For this review, take the finished solid that the model builds, in its own axes (mm). Face numbers are marked on the shaded views. A direction names the side the tool comes from. Give positions to 0.01 mm unless a question says otherwise; leave off trailing zeros. Loops run counter-clockwise (first coordinate to the right, second up) from the corner with the lowest first, then second, coordinate; pieces in that order, holes last. Notation, with made-up numbers: (36, -0.5) - (92, -0.5) arc R13 cw to (92, 20.5) - close; hole circle Ø8 at (-13.75, -2). An arc over 180 degrees is marked (long way). Answer as CSV lines item,"result".
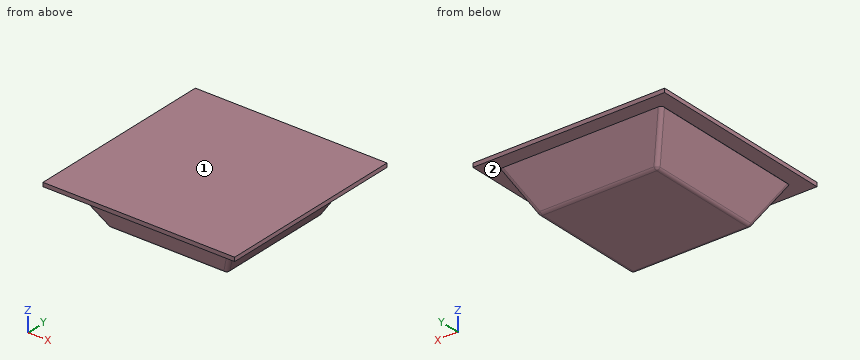
Solid Edge part; units mm, degrees
sketch "Sketch1" plane through (0, 0, 0) normal (0, 0, 1) x (1, 0, 0)
  line L0 (41, -41) -> (-41, -41)
  line L1 (-41, -41) -> (-41, 41)
  line L2 (-41, 41) -> (41, 41)
  line L3 (41, 41) -> (41, -41)
  dimension "D1" = 41
  dimension "D2" = 41
extrude "Protrusion1" add sketch "Sketch1" along normal blind 20
sketch "Sketch2" plane through (41, 0, 10) normal (1, 0, 0) x (0, 1, 0)
  line L0 (-41, 10) -> (-30, -10)
  line L1 (-30, -10) -> (30, -10)
  line L2 (30, -10) -> (41, 10)
  line L3 (-41, 10) -> (41, 10)
extrude "Cutout1" cut sketch "Sketch2" against normal through all flip side to cut
sketch "Sketch3" plane through (0, 0, 20) normal (0, 0, 1) x (0, 1, 0)
  line L0 (48.5, -48.5) -> (-48.5, -48.5)
  line L1 (-48.5, -48.5) -> (-48.5, 48.5)
  line L2 (-48.5, 48.5) -> (48.5, 48.5)
  line L3 (48.5, 48.5) -> (48.5, -48.5)
  dimension "D1" = 48.5
  dimension "D2" = 48.5
extrude "ExtrudedProtrusion_2" add sketch "Sketch3" along normal blind 2
sketch "Sketch4" plane through (0, -48.5, 21.5) normal (0, -1, 0) x (1, 0, 0)
  line L0 (41, -1.6) -> (30, -21.5)
  line L1 (30, -21.5) -> (-30, -21.5)
  line L2 (-30, -21.5) -> (-41, -1.6)
  line L3 (-41, -1.6) -> (-51.646, -1.6)
  line L4 (-51.646, -1.6) -> (-51.646, 3.6738)
  line L5 (-51.646, 3.6738) -> (52.1886, 3.6738)
  line L6 (52.1886, 3.6738) -> (52.1886, -1.6)
  line L7 (52.1886, -1.6) -> (41, -1.6)
  dimension "D1" = 30
extrude "Cutout2" cut sketch "Sketch4" against normal through all flip side to cut
fillet "Round_1" radius 2 8 edges at (-35.5, -35.4725, 9.95) (0, -30, 0) (-30, 0, 0) (-35.5, 35.4725, 9.95) (0, 30, 0) (35.5, 35.4725, 9.95) (30, 0, 0) (35.5, -35.4725, 9.95)
1) Consider section C-C on x = 42.5. Write out the cut boundary in (y, z), and give its area (3 significant figures).
From the geometry:
outline,"(-48.5, 20) - (48.5, 20) - (48.5, 22) - (-48.5, 22) - close"
area,"194 mm^2"
2) Wall thickness on line 1 (Z direction, x = 43.5, y = -1.5); line 2 (Z direction, x = 32, y = -4); line 3 (X direction, y = 25, z = 12.5): over which ranges is each line inside the solid? List them lowest first. Write a range as from..to.
From the geometry:
line 1,"z = 20..22"
line 2,"z = 3.62..22"
line 3,"x = -36.91..36.91"
3) Insertion check: P1, Ø1.5, axis at x = -29, z = 14.5, coming from the -Y side; P2, Ø4, axis at y = -2.5, z = 15, coming from the +X side; P3, Ø5, axis at x = 2.5, z = 13, coming from the +Y side (3 decimals); P4, Ø1.5, axis at x = -36, z = 8, coming from the -Y side. Each pin has a flat end and moves straight along its axis. Give the tip position at first contact, or say it passes through.
From the geometry:
P1,"stops at y = -38.39"
P2,"stops at x = 39.4"
P3,"stops at y = 38.525"
P4,"passes through"
4) Consider section B-B on x = -23. Write out the cut boundary in (y, z).
From the geometry:
outline,"(-48.5, 20) - (-41, 20) - (-30.57, 1.04) arc R2 ccw to (-28.82, 0) - (28.82, 0) arc R2 ccw to (30.57, 1.04) - (41, 20) - (48.5, 20) - (48.5, 22) - (-48.5, 22) - close"
5) Consider section A-A on y = 11. Write out the cut boundary in (x, z).
From the geometry:
outline,"(-48.5, 20) - (-41, 20) - (-41, 19.9) - (-30.57, 1.03) arc R2 ccw to (-28.82, 0) - (28.82, 0) arc R2 ccw to (30.57, 1.03) - (41, 19.9) - (41, 20) - (48.5, 20) - (48.5, 22) - (-48.5, 22) - close"
6) Machinability: for the marked faces 1 and 2, which of the approach directions +Z, -Z, +X, -X, +Y, -Y give a long, thin tool a straight path to every point of the face, cutting with its end or side? Answer none if there is none.
From the geometry:
face 1,"+Z, +X, -X, +Y, -Y"
face 2,"-Z"
